Part model, mm, in its own coordinate system. Coordinates: 2 decimals unless noted, no trailing zeros. Loops run counter-clockwise (first coordinate to the right, second up) from the corner with the lowest first, then second, coordinate; pieces in that order, holes last. Notation, with made-up numbers: M -29.5,-0.75 L -21.5,-0.75 A28 cw -21.5,26.25 Z; hole C -27.5,83.25 d7. An arc over 180 degrees is marked long. Answer as a JSON object with one key per item and string values. Group by question number.
1. Drill centre lines: L1, parallel to Y at x = -196.65, z = 0.45; L2, parallel to X at y = 16.5, z = 0.95 (3 decimals); L3, parallel to Y at x = 196.65, z = 0.3. Where is each one in solid material? Low to high.
2. Saw through at C-C on x = -101.5. Write the cut outline in (y, z), then the cut area to 3 significant figures.
3. Saw through at B-B on z = 0.6. Count the separate pieces of the cut face and the enclosed holes in it, then the cut area to 3 significant figures.
4. Saw through at A-A on x = 25.5. Write the cut outline in (y, z).
5. Drop flat-ended pins along their axis: pin 1 Ø1.5 at (x, z) = (197.5, 0.5) entering from +Y; pin 2 Ø1.5 at (y, z) = (33, -0.5) entering from +X; pin 3 Ø0.9 at (y, z) = (30.5, -0.5) entering from -X. Give the stop position or say it passes through.
from build123d import *

# Parameters (mm, degrees)
SKETCH1_W                  = 381
SKETCH1_H                  = 76.2
BOSS_EXTRUDE1_DEPTH        = 1.5
CUT_EXTRUDE1_DEPTH         = 195.29580541
SKETCH3_W                  = 15.875
SKETCH3_H                  = 12.7
BOSS_EXTRUDE2_DEPTH        = 3
FILLET1_R                  = 3.175
MIRROR1_START              = -1.5
MIRROR1_DEPTH              = 3
FILLET3_R                  = 1.5875
FILLET4_R                  = 3.175
F_8_CLEARANCE_HOLE1_D      = 4.4958
F_4_8_4_8_DIAMETER_HOLE1_D = 4.8
CUT_EXTRUDE2_DEPTH         = 210.883897965


# Read off the part's stored shape, not the designer's step: Mirror1
with BuildPart() as part:
    # Sketch1 → Boss-Extrude1 (new, symmetric)
    with BuildSketch(Plane.XY):
        Rectangle(SKETCH1_W, SKETCH1_H)
    extrude(amount=BOSS_EXTRUDE1_DEPTH, both=True)

    # Sketch5 → Cut-Extrude1 (cut, through all)
    with BuildSketch(Plane.XY.offset(1.5)):
        Polygon((-190.5, -38.1), (190.5, -4.766819197), (190.5, -38.1), align=None)
    extrude(amount=-CUT_EXTRUDE1_DEPTH, mode=Mode.SUBTRACT)

    # Sketch3 → Boss-Extrude2 (add)
    with BuildSketch(Plane.XY.offset(1.5)):
        with Locations((-198.4375, -19.05)):
            Rectangle(SKETCH3_W, SKETCH3_H)
        with Locations((198.4375, 16.666590402)):
            Rectangle(SKETCH3_W, SKETCH3_H)
    extrude(amount=-BOSS_EXTRUDE2_DEPTH)

    # Fillet1
    fillet1_edges = [part.edges().sort_by_distance(p)[0] for p in [
        (-206.375, -12.7, 0),
        (-206.375, -25.4, 0),
    ]]
    fillet(fillet1_edges, radius=FILLET1_R)

    # Mirror1 outline → Mirror1 (add)
    with BuildSketch(Plane.XY.offset(MIRROR1_START)):
        with BuildLine():
            Line((-206.375, 22.225), (-206.375, 15.875))
            ThreePointArc((-206.375, 15.875), (-205.44506403, 13.62993597), (-203.2, 12.7))
            Line((-203.2, 12.7), (-190.5, 12.7))
            Line((-190.5, 12.7), (-190.5, 25.4))
            Line((-190.5, 25.4), (-203.2, 25.4))
            ThreePointArc((-203.2, 25.4), (-205.44506403, 24.47006403), (-206.375, 22.225))
        make_face()
    extrude(amount=MIRROR1_DEPTH)

    # Fillet3
    fillet3_edges = [part.edges().sort_by_distance(p)[0] for p in [
        (190.5, 10.316590402, 0),
        (190.5, 23.016590402, 0),
        (-190.5, -25.4, 0),
        (-190.5, -12.7, 0),
        (-190.5, 25.4, 0),
        (-190.5, 12.7, 0),
    ]]
    fillet(fillet3_edges, radius=FILLET3_R)

    # Fillet4
    fillet4_edges = [part.edges().sort_by_distance(p)[0] for p in [
        (206.375, 23.016590402, 0),
        (206.375, 10.316590402, 0),
    ]]
    fillet(fillet4_edges, radius=FILLET4_R)

    # #8 Clearance Hole1 (through all)
    with Locations(Plane(origin=(0, 0, -1.5), x_dir=(-1, 0, 0), z_dir=(0, 0, -1))):
        with Locations((-46.681846327, 8.89), (-46.681846327, 27.432641431), (-90.478153673, 27.432641431), (-90.478153673, 8.89), (-106.1525, 33.896326852), (-122.0275, 33.896326852), (-122.0275, 5.321326852), (-106.1525, 5.321326852)):
            Hole(F_8_CLEARANCE_HOLE1_D / 2)

    # Ø4.8 (4.8) Diameter Hole1 (through all)
    with Locations(Plane.XY.offset(1.5)):
        with Locations((-196.65, 19.05), (-196.65, -19.05), (196.65, 16.666590402)):
            Hole(F_4_8_4_8_DIAMETER_HOLE1_D / 2)

    # Sketch12 → Cut-Extrude2 (cut, through all)
    with BuildSketch(Plane.XY.offset(1.5)):
        Polygon((190.5, -4.766819197), (165.1, -6.98903125), (190.5, 1.583180803), align=None)
    extrude(amount=-CUT_EXTRUDE2_DEPTH, mode=Mode.SUBTRACT)


solid = part.part
Outcome:
{
 "1": {"L1": "y = -25.4 to -21.45, -16.65 to -12.7, 12.7 to 16.65, 21.45 to 25.4", "L2": "x = -206.375 to 194.256, 199.044 to 206.375", "L3": "y = 10.32 to 14.27, 19.07 to 23.02"},
 "2": {"outline": "M -30.31,-1.5 L 38.1,-1.5 L 38.1,1.5 L -30.31,1.5 Z", "area": "205 mm²"},
 "3": {"separate pieces": "1", "enclosed holes": "11", "area": "23,000 mm²"},
 "4": {"outline": "M -19.2,-1.5 L 38.1,-1.5 L 38.1,1.5 L -19.2,1.5 Z"},
 "5": {"pin 1": "stops at y = 23.02", "pin 2": "stops at x = 190.5", "pin 3": "stops at x = -190.5"}
}
